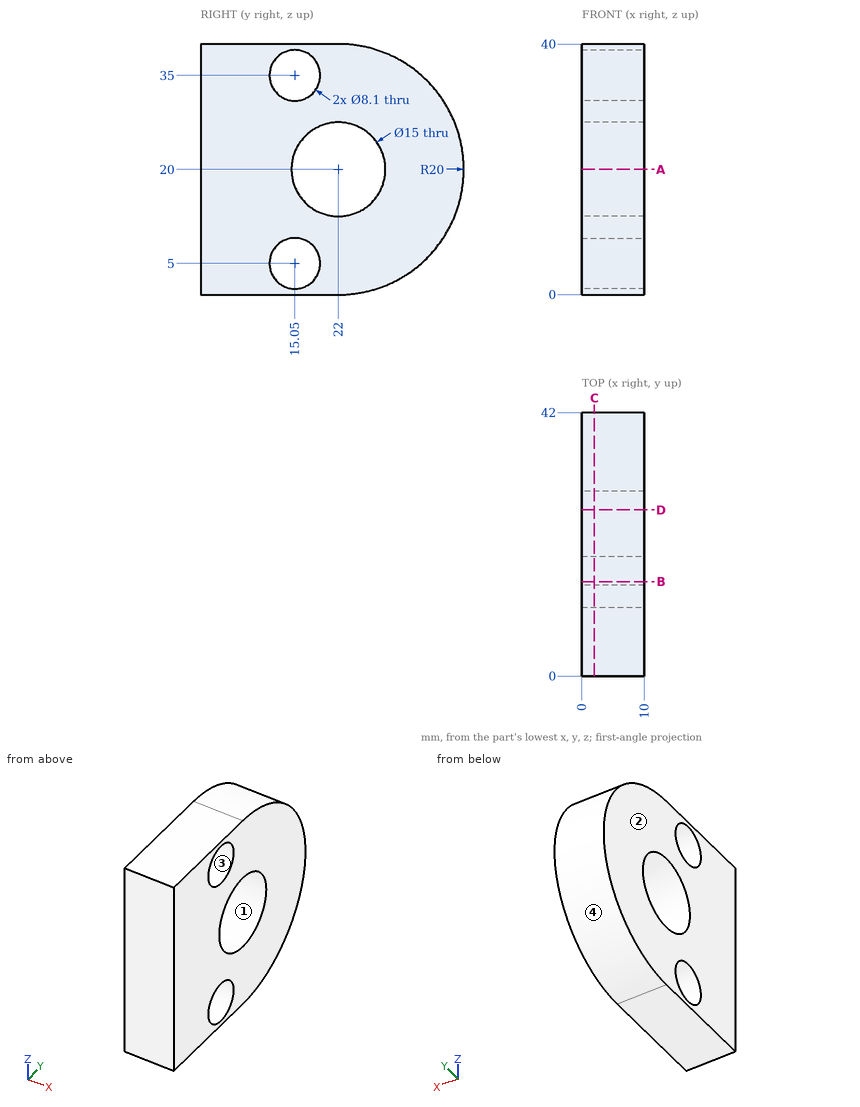
For this review, use the dimensioned drawing (mm, ordinates from the lowest corner) and the shaded views. Coordinates: 2 decimals unless noted, no trailing zeros. Write each loop counter-clockwise with the first axis right and the second up, starting at its lowest first coordinate (ties: lowest second). Pieces come first, ordered by that corner, then holes. Notation, with made-up numbers: (5, -5.5) -> (14, -5.5) arc R14 ccw to (14, 0.5) -> close; hole circle Ø3 at (-2, 2). An arc over 180 degrees is marked (long way). Write each question's results on one line, items separated by ' | '. Start each with the question number.
(1) Clearance check with flat-ended pins moving along their axes: P1, Ø3, axis at x = 5, z = 13.5, coming from the +Y side; P2, Ø4, axis at x = 6, z = 15, coming from the +Y side; P3, Ø1, axis at x = 3, z = 8.5, coming from the +Y side; P4, Ø13.5, axis at y = 22, z = 20, coming from the +X side. State where each tip first meets the part, or that it passes through.
(2) For line 1 along Z through (x, y) = (2.25, 22); line 2 along Z through (x, y) = (4.5, 13); line 3 along Y through (x, z) = (8, 36.5), list the stretches that pass through material, from the lowest coordinate up. Write a range as from..to.
(3) Take a section at D-D on y = 26.5. Write out the cut boundary in (x, z).
(4) Take a section at C-C on x = 2. Write out the cut boundary in (y, z).
(5) Take a section at B-B on y = 15.05. Write out the cut boundary in (x, z), and give its area (3 significant figures).
(6) The part is to be moulded in two halves that separate along Y. For the marked faces 1, 2, 3 and 4, say which applies: pulls with the +Y half, pulls with the -Y half, needs draft (parallel to the pull), parting line crosses it, or undercut.
(7) Take a section at A-A on z = 20. Write out the cut boundary in (x, y).
Results found:
1) P1: stops at y = 41.36 | P2: stops at y = 41.77 | P3: stops at y = 38.7 | P4: passes through
2) line 1: z = 0..12.5, 27.5..40 | line 2: z = 0..1.51, 8.49..31.51, 38.49..40 | line 3: y = 0..11.29, 18.81..33.3
3) outline: (0, 0.51) -> (10, 0.51) -> (10, 14) -> (0, 14) -> close; (0, 26) -> (10, 26) -> (10, 39.49) -> (0, 39.49) -> close
4) outline: (0, 0) -> (22, 0) arc R20 ccw to (22, 40) -> (0, 40) -> close; hole circle Ø8.1 at (15.05, 5); hole circle Ø8.1 at (15.05, 35); hole circle Ø15 at (22, 20)
5) outline: (0, 0) -> (10, 0) -> (10, 0.95) -> (0, 0.95) -> close; (0, 9.05) -> (10, 9.05) -> (10, 17.18) -> (0, 17.18) -> close; (0, 22.82) -> (10, 22.82) -> (10, 30.95) -> (0, 30.95) -> close; (0, 39.05) -> (10, 39.05) -> (10, 40) -> (0, 40) -> close | area: 182 mm2
6) face 1: undercut | face 2: needs draft | face 3: undercut | face 4: pulls with the +Y half
7) outline: (0, 0) -> (10, 0) -> (10, 14.5) -> (0, 14.5) -> close; (0, 29.5) -> (10, 29.5) -> (10, 42) -> (0, 42) -> close
